Autodesk Inventor part; units mm, degrees
ref_plane "YZ Plane" through (0, 0, 0) normal (1, 0, 0) x (0, 1, 0)
ref_plane "XZ Plane" through (0, 0, 0) normal (0, 1, 0) x (-1, 0, 0)
ref_plane "XY Plane" through (0, 0, 0) normal (0, 0, 1) x (1, 0, 0)
sketch "Sketch1" plane through (0, 0, 0) normal (0, 1, 0) x (-1, 0, 0)
  line L0 (0, 2) -> (5, 2)
  line L1 (5, 2) -> (5, -16)
  line L2 (0, -20) -> (0, 2)
  line L3 (0, -44) -> (5, -44)
  line L4 (5, -44) -> (5, -33.4641)
  arc A0 (13, -29) -> (5, -29) centre (9, -29) ccw
  line L5 (9, -20) -> (14, -20)
  line L6 (18, -44) -> (13, -44)
  line L7 (13, -44) -> (13, -33.4641)
  line L8 (18, -24) -> (18, -44)
  line L9 (0, -20) -> (0, -44)
  arc A1 (5, -16) -> (9, -20) centre (9, -16) ccw
  arc A2 (18, -24) -> (14, -20) centre (14, -24) ccw
  circle A3 centre (9, -29) radius 4 construction
  line L10 (6, -32.4641) -> (6.2193, -32.4641)
  line L11 (12, -32.4641) -> (11.7807, -32.4641)
  arc A4 (5, -29) -> (6.3829, -32.025) centre (9, -29) ccw
  arc A5 (11.6171, -32.025) -> (13, -29) centre (9, -29) ccw
  arc A6 (6.2193, -32.4641) -> (6.3829, -32.025) centre (6.2193, -32.2141) ccw
  arc A7 (11.6171, -32.025) -> (11.7807, -32.4641) centre (11.7807, -32.2141) ccw
  arc A8 (6, -32.4641) -> (5, -33.4641) centre (6, -33.4641) ccw
  arc A9 (13, -33.4641) -> (12, -32.4641) centre (12, -33.4641) ccw
  point P0 (0, 0)
  point P1 (7, -32.4641)
  point P2 (11, -32.4641)
  dimension "d45" = 1
extrude "Extrusion1" add sketch "Sketch1" along normal blind 10
move or copy body "Move Body1" bodies to move or copy 1 copy no rotation origin (0, 0, 0) rotation axis (1, 0, 0) rotation angle -90 translate (0, 54, -34)
sketch "Sketch4" plane through (0, 10, -34) normal (1, 0, 0) x (0, 0, -1)
  line L0 (0, 46) -> (10, 46) construction
  line L1 (5, 46) -> (5, 41) construction
  circle A0 centre (5, 41) radius 2
  circle A1 centre (5, 31.5) radius 2
  circle A2 centre (5, 5) radius 2
  dimension "d29" = 5
  dimension "d30" = 4
  dimension "d31" = 4
  dimension "d32" = 4
extrude "Extrusion3" cut sketch "Sketch4" against normal blind 5
sketch "Sketch5" plane through (0, 10, -34) normal (1, 0, 0) x (0, 0, -1)
  circle A0 centre (5, 5) radius 2 construction
  circle A1 centre (5, 5) radius 3.25 construction
  line L0 (8.25, 5) -> (6.625, 2.1854)
  line L1 (6.625, 2.1854) -> (3.375, 2.1854)
  line L2 (3.375, 2.1854) -> (1.75, 5)
  line L3 (1.75, 5) -> (3.375, 7.8146)
  line L4 (3.375, 7.8146) -> (6.625, 7.8146)
  line L5 (6.625, 7.8146) -> (8.25, 5)
  point P0 (-34, -10)
  dimension "d35" = 6.5
extrude "Extrusion4" cut sketch "Sketch5" against normal blind 2.5
sketch "Sketch6" plane through (-18, 10, -34) normal (-1, 0, 0) x (0, 0, 1)
  line L0 (0, 0) -> (-10, 0) construction
  line L1 (-5, 0) -> (-5, 5) construction
  circle A0 centre (-5, 5) radius 2
  point P0 (34, -10)
  dimension "d38" = 5
  dimension "d39" = 4
extrude "Extrusion5" cut sketch "Sketch6" against normal blind 5
properties part number "Camera_Bed_Detector"
Model file for the job. Use its own axes, mm. A direction names the side the tool comes from. Give positions to 0.01 mm unless a question says otherwise; leave off trailing zeros. Order: outer loops, then holes, each group sorted by start corner. A loop starts at its lowest first (then second) coordinate and runs counter-clockwise, first axis right, second up.
1) Mould opens along Y. For faces 4 (the cylindrical face through (-15.535, 16.352, -40.474)), 5 (the flat face through (-11, 34, -39)), 6 (the flat face through (-18, 20, -39)) say: +Y half, -Y half, draft (parallel to the pull), parting line (faces both ways), or undercut.
2) Saw through at A-A, the plane y = 51. Write the cut outline in (x, z).
3) 3-axis set-ups, long thin cutter, end or side, ignore diameter. For faces 1 (the flat face through (-5, 15.2, -36.7)), 2 (the flat face through (-5, 47, -39)), 3 (the flat face through (-1.232, 13.612, -41.449)): which of +Z, -Z, +X, -X, +Y, -Y reach the whole face in a straight line?
4) Wall check: probe 1 along Y at (x, z) = (-4.4, -39); probe 2 along Y at (x, z) = (-2.4, -39); probe 3 along X at (y, z) = (19, -35.25). Give the ranges that are in metal, low to high.
5) Saw through at B-B, the plane x = -4. Write the cut outline in (y, z).
6) Saw through at D-D, the plane x = -14.5. Write the cut outline in (y, z).
7) Saw through at C-C, the plane z = -35. Write the cut outline in (x, y) (3 decimals), then the cut area to 3 significant figures.
8) Pin check, flat tips, straight feed: pin 1 (4.5 mm diameter, centred on y = 15, z = -39, fed in from +X); pin 2 (2 mm diameter, centred on x = -6.5, z = -37.5, fed in from +Y); pin 3 (5.5 mm diameter, centred on x = -11, z = -39.5, fed in from +Y). Stop position of each tip, or through.
Computed:
1. face 4: undercut
1. face 5: +Y half
1. face 6: draft
2. outline: (-5, -44) - (0, -44) - (0, -41) - (-5, -41) - close; (-5, -37) - (0, -37) - (0, -34) - (-5, -34) - close
3. face 1: +Z, -Z, -Y
3. face 2: +Z, -Z, -X, +Y
3. face 3: +X
4. probe 1: y = 10 to 13, 17 to 39.5, 43.5 to 49, 53 to 56
4. probe 2: y = 10 to 12.19, 17.81 to 39.5, 43.5 to 49, 53 to 56
4. probe 3: x = -18 to -13, -5 to 0
5. outline: (10, -44) - (56, -44) - (56, -34) - (10, -34) - close; hole circle Ø4 at (15, -39); hole circle Ø4 at (41.5, -39); hole circle Ø4 at (51, -39)
6. outline: (10, -44) - (33.97, -44) - (33.97, -34) - (10, -34) - close; hole circle Ø4 at (15, -39)
7. outline: (-18, 10) - (-13, 10) - (-13, 20.536) arc R1 cw to (-12, 21.536) - (-11.781, 21.536) arc R0.25 ccw to (-11.617, 21.975) arc R4 cw to (-13, 25) arc R4 cw to (-5, 25) arc R4 cw to (-6.383, 21.975) arc R0.25 ccw to (-6.219, 21.536) - (-6, 21.536) arc R1 cw to (-5, 20.536) - (-5, 10) - (0, 10) - (0, 56) - (-5, 56) - (-5, 38) arc R4 cw to (-9, 34) - (-14, 34) arc R4 ccw to (-18, 30) - close
7. area: 401 mm2
8. pin 1: stops at x = -2.5
8. pin 2: stops at y = 36.06
8. pin 3: stops at y = 34.07
